Source: CAD feature listing. Evaluate the final solid. Frame: model axes, mm. Coordinates: 2 decimals unless noted, no trailing zeros. Order: outer loops, then holes, each group sorted by start corner. A loop starts at its lowest first (then second) coordinate and runs counter-clockwise, first axis right, second up. Notation, with made-up numbers: (-38, 6) - (-13, 6) arc R28 ccw to (-13, 26) - close; hole circle Ø7 at (21.25, -8). An arc over 180 degrees is marked (long way). One line per question, with ' | ' between items. Start each with the question number.
(1) Section C-C (z = 2.1). Count the separate pieces of the cut face and the enclosed holes in it, then the cut area to 3 significant figures.
(2) Draft query along Y for faces 1 (the flat face through (12, 0, 3.302)), 2 (the cylindrical face through (0.17, 19.05, 1.63)), 3 (the cylindrical face through (26.35, -0.11, 1.63)), 4 (the cylindrical face through (-17.24, -0.55, 1.63)). Return one class per face: +Y half, -Y half, draft (parallel to the pull), parting line (faces both ways), or undercut.
(3) Contact query for flat-ended pins moving along their axis: P1, Ø1.5, axis at x = -19.5, z = 1, coming from the -Y side; P2, Ø3.5, axis at x = 10.96, y = -10.96, coming from the +Z side; P3, Ø4, axis at x = 0, y = 15.494, coming from the +Z side. Output: stop coordinate, or through.
(4) Section A-A (x = 0). Return the cut outline in (y, z), then the cut area to 3 significant figures.
(5) Section D-D (y = -7). Return the cut outline in (x, z), then the cut area to 3 significant figures.
(6) Line query: line 1 along Y through (x, z) = (0, 2.3); line 2 along X through (y, z) = (6, 1.6); line 3 along X through (y, z) = (10, 0.6) (3 decimals). Output: solid intervals per line, ascending.
(7) Section B-B (y = 0). Return the cut outline in (x, z) (1 decimal).
from build123d import *

# Parameters (mm, degrees)
SKETCH1_R           = 11.112500335
SKETCH1_R_2         = 1.828800055
SKETCH1_R_3         = 2.489200075
SKETCH1_R_4         = 2.540000076
BOSS_EXTRUDE1_DEPTH = 3.302


with BuildPart() as part:
    # Sketch1 → Boss-Extrude1 (new body)
    with BuildSketch(Plane.XY):
        with BuildLine():
            Line((-26.670000803, -3.810000115), (-11.430000344, -15.240000459))
            ThreePointArc((-11.430000344, -15.240000459), (0, -19.050000574), (11.430000344, -15.240000459))
            Line((11.430000344, -15.240000459), (26.670000803, -3.810000115))
            ThreePointArc((26.670000803, -3.810000115), (28.57500086, 0), (26.670000803, 3.810000115))
            Line((26.670000803, 3.810000115), (11.430000344, 15.240000459))
            ThreePointArc((11.430000344, 15.240000459), (0, 19.050000574), (-11.430000344, 15.240000459))
            Line((-11.430000344, 15.240000459), (-26.670000803, 3.810000115))
            ThreePointArc((-26.670000803, 3.810000115), (-28.57500086, 0), (-26.670000803, -3.810000115))
        make_face()
        with Locations(Location((0, 0, 0), (0, 0, 180))):
            Circle(SKETCH1_R, mode=Mode.SUBTRACT)
        with Locations(Location((0, 15.494000466, 0), (0, 0, 180))):
            Circle(SKETCH1_R_2, mode=Mode.SUBTRACT)
        with Locations(Location((-15.494000466, 0, 0), (0, 0, 180))):
            Circle(SKETCH1_R_2, mode=Mode.SUBTRACT)
        with Locations(Location((-14.314589908, 5.92929728, 0), (0, 0, 180))):
            Circle(SKETCH1_R_2, mode=Mode.SUBTRACT)
        with Locations(Location((-5.92929728, 14.314589908, 0), (0, 0, 180))):
            Circle(SKETCH1_R_2, mode=Mode.SUBTRACT)
        with Locations(Location((-10.955912798, 10.955912798, 0), (0, 0, 180))):
            Circle(SKETCH1_R_2, mode=Mode.SUBTRACT)
        with Locations(Location((0, -15.494000466, 0), (0, 0, 180))):
            Circle(SKETCH1_R_2, mode=Mode.SUBTRACT)
        with Locations(Location((15.494000466, 0, 0), (0, 0, 180))):
            Circle(SKETCH1_R_2, mode=Mode.SUBTRACT)
        with Locations(Location((14.314589908, -5.92929728, 0), (0, 0, 180))):
            Circle(SKETCH1_R_2, mode=Mode.SUBTRACT)
        with Locations(Location((5.92929728, -14.314589908, 0), (0, 0, 180))):
            Circle(SKETCH1_R_2, mode=Mode.SUBTRACT)
        with Locations(Location((10.955912798, -10.955912798, 0), (0, 0, 180))):
            Circle(SKETCH1_R_2, mode=Mode.SUBTRACT)
        with Locations(Location((-23.812500717, 0, 0), (0, 0, 180))):
            Circle(SKETCH1_R_3, mode=Mode.SUBTRACT)
        with Locations(Location((23.812500717, 0, 0), (0, 0, 180))):
            Circle(SKETCH1_R_4, mode=Mode.SUBTRACT)
    extrude(amount=BOSS_EXTRUDE1_DEPTH)


solid = part.part
Response values:
1) separate pieces: 1 | enclosed holes: 13 | area: 884 mm²
2) face 1: draft | face 2: +Y half | face 3: undercut | face 4: undercut
3) P1: stops at y = -9.75 | P2: passes through | P3: stops at z = 3.3
4) outline: (-19.05, 0) - (-17.32, 0) - (-17.32, 3.3) - (-19.05, 3.3) - close; (-13.67, 0) - (-11.11, 0) - (-11.11, 3.3) - (-13.67, 3.3) - close; (11.11, 0) - (13.67, 0) - (13.67, 3.3) - (11.11, 3.3) - close; (17.32, 0) - (19.05, 0) - (19.05, 3.3) - (17.32, 3.3) - close | area: 28.3 mm²
5) outline: (-22.42, 0) - (-8.63, 0) - (-8.63, 3.3) - (-22.42, 3.3) - close; (8.63, 0) - (12.83, 0) - (12.83, 3.3) - (8.63, 3.3) - close; (15.8, 0) - (22.42, 0) - (22.42, 3.3) - (15.8, 3.3) - close | area: 81.3 mm²
6) line 1: y = -19.05 to -17.32, -13.67 to -11.11, 11.11 to 13.67, 17.32 to 19.05 | line 2: x = -23.75 to -16.14, -12.49 to -9.35, 9.35 to 23.75 | line 3: x = -18.417 to -12.515, -9.397 to -4.846, 4.846 to 18.417
7) outline: (-28.6, 0) - (-26.3, 0) - (-26.3, 3.3) - (-28.6, 3.3) - close; (-21.3, 0) - (-17.3, 0) - (-17.3, 3.3) - (-21.3, 3.3) - close; (-13.7, 0) - (-11.1, 0) - (-11.1, 3.3) - (-13.7, 3.3) - close; (11.1, 0) - (13.7, 0) - (13.7, 3.3) - (11.1, 3.3) - close; (17.3, 0) - (21.3, 0) - (21.3, 3.3) - (17.3, 3.3) - close; (26.4, 0) - (28.6, 0) - (28.6, 3.3) - (26.4, 3.3) - close
